Part model, mm, in its own coordinate system. A direction names the side the tool comes from. Give positions to 0.01 mm unless a question says otherwise; leave off trailing zeros. Order: outer loops, then holes, each group sorted by start corner. A loop starts at its lowest first (then second) coordinate and runs counter-clockwise, first axis right, second up. Notation, with made-up numbers: (-26, 83) - (20, 83) arc R25 cw to (20, 101) - close; hole circle Ø9 at (39.25, -35). An arc over 180 degrees is marked (long way). One line per item, written item: value.
```python
from build123d import *

# Parameters (mm, degrees)
SKETCH1_W               = 53.98
SKETCH1_H               = 1.59
BOSS_EXTRUDE1_DEPTH     = 20.64
SKETCH1_3_W             = 53.98
SKETCH1_3_H             = 18.26
SKETCH1_3_R             = 3.175
SKETCH1_3_H_2           = 18.25
BOSS_EXTRUDE2_DEPTH     = 1.59
CUT_EXTRUDE1_DEPTH      = 39.134827914
CUT_EXTRUDE1_DEPTH_BACK = 39.134827914
SKETCH3_W               = 53.98
SKETCH3_H               = 18.26


with BuildPart() as part:
    # Sketch1 → Boss-Extrude1 (new body)
    with BuildSketch(Plane(origin=(0, 0, 0), x_dir=(1, 0, 0), z_dir=(0, 1, 0))):
        with Locations((0, 0.005)):
            Rectangle(SKETCH1_W, SKETCH1_H)
    extrude(amount=BOSS_EXTRUDE1_DEPTH)

    # Sketch1_3 → Boss-Extrude2 (add)
    # profile 1 of 2: a face of its own
    with BuildSketch(Plane(origin=(0, 0, 0), x_dir=(1, 0, 0), z_dir=(0, 1, 0))):
        with Locations((0, -9.92)):
            Rectangle(SKETCH1_3_W, SKETCH1_3_H)
        with Locations(Location((-13.825, -10.08, 0), (0, 0, 90))):
            Circle(SKETCH1_3_R, mode=Mode.SUBTRACT)
        with Locations(Location((13.825, -10.08, 0), (0, 0, 90))):
            Circle(SKETCH1_3_R, mode=Mode.SUBTRACT)
    # profile 2 of 2: a face of its own
    with BuildSketch(Plane(origin=(0, 0, 0), x_dir=(1, 0, 0), z_dir=(0, 1, 0))):
        with Locations((0, 9.925)):
            Rectangle(SKETCH1_3_W, SKETCH1_3_H_2)
        with Locations(Location((-13.825, 10.08, 0), (0, 0, 90))):
            Circle(SKETCH1_3_R, mode=Mode.SUBTRACT)
        with Locations(Location((13.825, 10.08, 0), (0, 0, 90))):
            Circle(SKETCH1_3_R, mode=Mode.SUBTRACT)
    extrude(amount=BOSS_EXTRUDE2_DEPTH)

    # Sketch3 → Cut-Extrude1 (cut, two sides: drawn at the far end of the back side and taken through both)
    with BuildSketch(Plane(origin=(0, 1.59, 0), x_dir=(1, 0, 0), z_dir=(0, 1, 0)).offset(-CUT_EXTRUDE1_DEPTH_BACK)):
        with Locations((0, -9.92)):
            Rectangle(SKETCH3_W, SKETCH3_H)
    extrude(amount=CUT_EXTRUDE1_DEPTH + CUT_EXTRUDE1_DEPTH_BACK, mode=Mode.SUBTRACT)


solid = part.part
```
1) Which spindle directions (+Z, -Z, +X, -X, +Y, -Y) get a long thin tool onto all of the face, cutting with end or side? Do faces 1 (the cylindrical face through (-11.893, 0.784, -7.56)), 2 (the flat face through (0, 11, -0.8)). Say none if no direction does.
Outcome:
face 1: +Y, -Y
face 2: -Z, +X, -X, +Y
2) Mould opens along X. For faces 3 (the flat face through (-26.99, 6, 0)), 4 (the flat face through (0, 20.64, 0)), 5 (the cylindrical face through (15.757, 0.784, -7.56)) say: released by +X, released by -X, zero draft, split by the parting line, or undercut.
Outcome:
face 3: released by -X
face 4: zero draft
face 5: undercut
3) Cut at A-A, the plane z = -10.08. Give the cut face in (x, y).
Outcome:
outline: (-26.99, 0) - (-17, 0) - (-17, 1.59) - (-26.99, 1.59) - close; (-10.65, 0) - (10.65, 0) - (10.65, 1.59) - (-10.65, 1.59) - close; (17, 0) - (26.99, 0) - (26.99, 1.59) - (17, 1.59) - close
4) Cut at D-D, the plane z = -12.5. Give the cut face in (x, y).
Outcome:
outline: (-26.99, 0) - (-15.88, 0) - (-15.88, 1.59) - (-26.99, 1.59) - close; (-11.77, 0) - (11.77, 0) - (11.77, 1.59) - (-11.77, 1.59) - close; (15.88, 0) - (26.99, 0) - (26.99, 1.59) - (15.88, 1.59) - close
5) Cut at B-B, the plane x = 1. Give the cut face in (y, z).
Outcome:
outline: (0, -19.05) - (1.59, -19.05) - (1.59, -0.8) - (20.64, -0.8) - (20.64, 0.79) - (0, 0.79) - close
6) Pin check, flat tips, straight feed: pin 1 (4 mm diameter, centred on x = 13.825, z = -10.08, fed in from -Y); pin 2 (10 mm diameter, centred on x = 15, y = 17, fed in from -Z); pin 3 (9 mm diameter, centred on x = -10, z = -13, fed in from +Y). Stop position of each tip, or through.
Outcome:
pin 1: passes through
pin 2: stops at z = -0.8
pin 3: stops at y = 1.59
7) Cut at C-C, the plane y = 7.5. Give the cut face in (x, z).
Outcome:
outline: (-26.99, -0.8) - (26.99, -0.8) - (26.99, 0.79) - (-26.99, 0.79) - close
8) Drill centre lines: line 1 along X through (y, z) = (0.45, -10.08); line 2 along Y through (x, z) = (0.5, -17.5); line 3 along Z through (x, y) = (2.5, 15.75). Where is each one in solid material? Low to high. Write a range as from..to.
Outcome:
line 1: x = -26.99..-17, -10.65..10.65, 17..26.99
line 2: y = 0..1.59
line 3: z = -0.8..0.79
